Check sheet for the drawn part. Datum: minimum x, y, z corner. Units: mm. Give positions to 0.01 mm unless a question says otherwise; leave off trailing zeros. Write each loop counter-clockwise with the first axis right and the second up, starting at its lowest first coordinate (ties: lowest second). Pieces come first, ordered by that corner, then holes.
(1) Cross-section at C-C (x = 36). Record the boundary of the cut face in (y, z).
(2) Cross-section at D-D (y = 10.5). Record the boundary of the cut face in (x, z).
(3) Depth check by flat-ended pin: P1, Ø12, axis at x = 8.5, y = 25.5, coming from the +Z side. Enter the tip coordinate at first touch or a pass-through.
(4) Thickness scan on line 1 along Z through (x, y) = (19.5, 8.5); line 2 along X through (y, z) = (23, 4.5). Record the ranges inside material, lowest first.
(5) Cross-section at A-A (x = 67). Record the boundary of the cut face in (y, z).
(6) Cross-section at B-B (y = 21.5). Record the boundary of the cut face in (x, z).
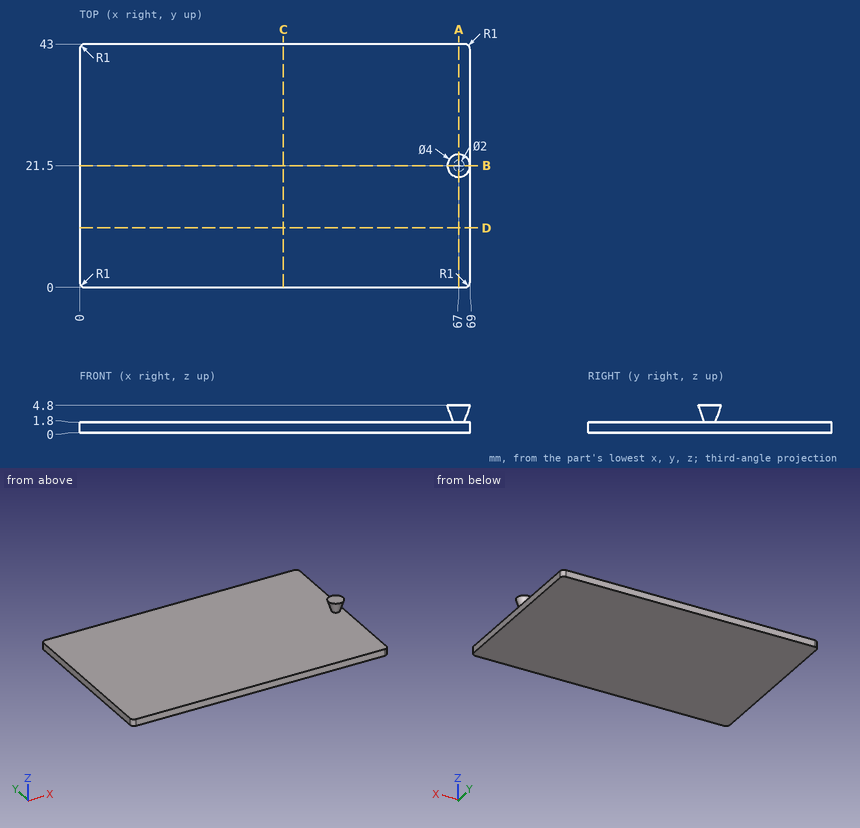
Reply:
1. outline: (0, 0) - (43, 0) - (43, 1.8) - (0, 1.8) - close
2. outline: (0, 0) - (69, 0) - (69, 1.8) - (0, 1.8) - close
3. P1: stops at z = 1.8
4. line 1: z = 0 to 1.8
4. line 2: x = 65.83 to 68.17
5. outline: (0, 0) - (43, 0) - (43, 1.8) - (22.5, 1.8) - (23.5, 4.8) - (19.5, 4.8) - (20.5, 1.8) - (0, 1.8) - close
6. outline: (0, 0) - (69, 0) - (69, 1.8) - (68, 1.8) - (69, 4.8) - (65, 4.8) - (66, 1.8) - (0, 1.8) - close
